from build123d import *

# Parameters (mm, degrees)
SKETCH1_R           = 25.4
BOSS_EXTRUDE1_DEPTH = 101.6
SKETCH8_W           = 25.4
SKETCH8_H           = 76.2
BOSS_EXTRUDE2_DEPTH = 76.2
SKETCH9_R           = 13.092802434
BOSS_EXTRUDE3_DEPTH = 0.254
DOME1_FACE_RADIUS   = 13.092802434
DOME1_HEIGHT        = 2.38
SKETCH10_R          = 12.541774092
BOSS_EXTRUDE4_DEPTH = 0.254


# Read off the part's stored shape, not the designer's step: Dome2
with BuildPart() as part:
    # Sketch1 → Boss-Extrude1 (new, symmetric)
    with BuildSketch(Plane.XY):
        Circle(SKETCH1_R)
    extrude(amount=BOSS_EXTRUDE1_DEPTH, both=True)

    # Sketch8 → Boss-Extrude2 (add)
    with BuildSketch(Plane(origin=(38.1, 0, 0), x_dir=(0, 0, -1), z_dir=(1, 0, 0))):
        with Locations((-63.5, 0)):
            Rectangle(SKETCH8_W, SKETCH8_H)
    extrude(amount=-BOSS_EXTRUDE2_DEPTH)

    # Mirror1: part across plane


with BuildPart() as part_1:
    add(part.part)
    add(part.part.mirror(Plane.XY))

    # Sketch9 → Boss-Extrude3 (add)
    with BuildSketch(Plane.XY.offset(101.6)):
        Circle(SKETCH9_R)
    extrude(amount=BOSS_EXTRUDE3_DEPTH)

    # Dome1: a dome of height H over a round flat face of radius A is a cap of a sphere of radius (A * A + H * H) / (2 * H)
    dome1_r = (DOME1_FACE_RADIUS * DOME1_FACE_RADIUS + DOME1_HEIGHT * DOME1_HEIGHT) / (2 * DOME1_HEIGHT)
    dome1_base = Plane((0, 0, 101.854), z_dir=(0, 0, 1))
    with Locations(dome1_base.offset(DOME1_HEIGHT - dome1_r)):
        dome1_ball = Sphere(dome1_r, mode=Mode.PRIVATE)
    add(split(dome1_ball, bisect_by=dome1_base, keep=Keep.TOP, mode=Mode.PRIVATE))

    # Sketch10 → Boss-Extrude4 (add)
    with BuildSketch(Plane(origin=(0, 0, -101.6), x_dir=(-1, 0, 0), z_dir=(0, 0, -1))):
        Circle(SKETCH10_R)
    extrude(amount=BOSS_EXTRUDE4_DEPTH)

    # Dome2 outline → Dome2 (revolve)
    with BuildSketch(Plane.XZ):
        with BuildLine():
            Line((0, -101.853999987), (0, -104.234))
            ThreePointArc((0, -104.234), (6.382799116, -103.633737683), (12.541774124, -101.853999987))
            Line((12.541774124, -101.853999987), (0, -101.853999987))
        make_face()
    revolve(axis=Axis((0, 0, 0), (0, 0, 1)))


solid = part_1.part
Part model, mm, in its own coordinate system. A direction names the side the tool comes from. Coordinates: 2 decimals unless noted, no trailing zeros. Loops run counter-clockwise (first coordinate to the right, second up) from the corner with the lowest first, then second, coordinate; pieces in that order, holes last. Notation, with made-up numbers: M 60,-21.5 L 81,-21.5 A16 ccw 81,-6.5 Z; hole C -5.75,-5.5 d3. An arc over 180 degrees is marked long. Use a Markdown table: item, result. Add a question column.
Q1. Cut at D-D (y = 9.5). Write the cut outline in (x, z).
Q2. Cut at A-A (y = 0). Write the cut outline in (x, z), and give its area (3 significant figures).
Q3. Which spindle directions (+Z, -Z, +X, -X, +Y, -Y) get a long thin tool onto all of the face, cutting with end or side? Do faces 5 (the cylindrical face through (-5.506, -24.796, 0.711)), 6 (the cylindrical face through (-5.506, -24.796, 89.078)), 7 (the cylindrical face through (-5.506, -24.796, -88.722)), 8 (the flat face through (1, -38.1, -64)). Say none if no direction does.
Q4. Cut at C-C (z = -29). Write the cut outline in (x, y).
Q5. Mould opens along Z. For faces 1 (the flat face through (-38.1, 1, -64)), 2 (the flat face through (26, -1, -50.8)), 3 (the flat face through (26, -1, 50.8)), 4 (the flat face through (26, -1, 76.2)) say: +Z half, -Z half, draft (parallel to the pull), parting line (faces both ways), or undercut.
Q6. Probe L1, parallel to Z at x = -25, y = 27; L2, parallel to Z at x = -20, y = -15.5; L3, parallel to X at y = 0.5, z = -19. List the from-to ranges inside material, lowest first.
Q7. Pin check, flat tips, straight feed: P1, Ø2, axis at x = 7, y = 14, coming from the -Z side; P2, Ø1, axis at x = 26.5, y = -5, coming from the +Z side; P3, Ø8, axis at x = 9, z = -40, coming from the -Y side. Stop position of each tip, or through.
Worked out:
| question | item | result |
|---|---|---|
| 1 | outline | M -38.1,-76.2 L -23.56,-76.2 L -23.56,-101.6 L -8.19,-101.6 L -8.19,-101.85 A32.89 ccw 8.19,-101.85 L 8.19,-101.6 L 23.56,-101.6 L 23.56,-76.2 L 38.1,-76.2 L 38.1,-50.8 L 23.56,-50.8 L 23.56,50.8 L 38.1,50.8 L 38.1,76.2 L 23.56,76.2 L 23.56,101.6 L 9.01,101.6 L 9.01,101.85 A35.97 ccw -9.01,101.85 L -9.01,101.6 L -23.56,101.6 L -23.56,76.2 L -38.1,76.2 L -38.1,50.8 L -23.56,50.8 L -23.56,-50.8 L -38.1,-50.8 Z |
| 2 | outline | M -38.1,-76.2 L -25.4,-76.2 L -25.4,-101.6 L -12.54,-101.6 L -12.54,-101.85 A34.24 ccw 12.54,-101.85 L 12.54,-101.6 L 25.4,-101.6 L 25.4,-76.2 L 38.1,-76.2 L 38.1,-50.8 L 25.4,-50.8 L 25.4,50.8 L 38.1,50.8 L 38.1,76.2 L 25.4,76.2 L 25.4,101.6 L 13.09,101.6 L 13.09,101.85 A37.2 ccw -13.09,101.85 L -13.09,101.6 L -25.4,101.6 L -25.4,76.2 L -38.1,76.2 L -38.1,50.8 L -25.4,50.8 L -25.4,-50.8 L -38.1,-50.8 Z |
| 2 | area | 11,700 mm2 |
| 3 | face 5 | none |
| 3 | face 6 | +Z |
| 3 | face 7 | -Z |
| 3 | face 8 | +Z, -Z, +X, -X, -Y |
| 4 | outline | C 0,0 d50.8 |
| 5 | face 1 | draft |
| 5 | face 2 | undercut |
| 5 | face 3 | undercut |
| 5 | face 4 | +Z half |
| 6 | L1 | z = -76.2 to -50.8, 50.8 to 76.2 |
| 6 | L2 | z = -101.6 to 101.6 |
| 6 | L3 | x = -25.4 to 25.4 |
| 7 | P1 | stops at z = -101.6 |
| 7 | P2 | stops at z = 76.2 |
| 7 | P3 | stops at y = -24.9 |
